Part print with two shaded views. Sizes in mm from the minimum x, y, z corner. Round coordinates to 2 decimals unless told otherwise and drop trailing zeros. Order: outer loops, then holes, each group sorted by start corner. A loop starts at its lowest first (then second) coordinate and runs counter-clockwise, first axis right, second up. Notation, with made-up numbers: M 61,76.5 L 97,76.5 A3 cw 97,81.5 Z; hole C 46,62 d10. An arc over 180 degrees is marked long. Return JSON: item names as keys, results as strings. Group by question number.
Item 1: Slice it at A-A on x = 18. Write the cut outline in (y, z).
Item 2: Slice it at D-D on z = 37. Write the cut outline in (x, y).
Item 3: Probe line 1 along X through (y, z) = (0.1, 21); line 2 along Z through (x, y) = (9.5, 0.2); line 3 along X through (y, z) = (0.3, 11). List the from-to ranges inside material, lowest first.
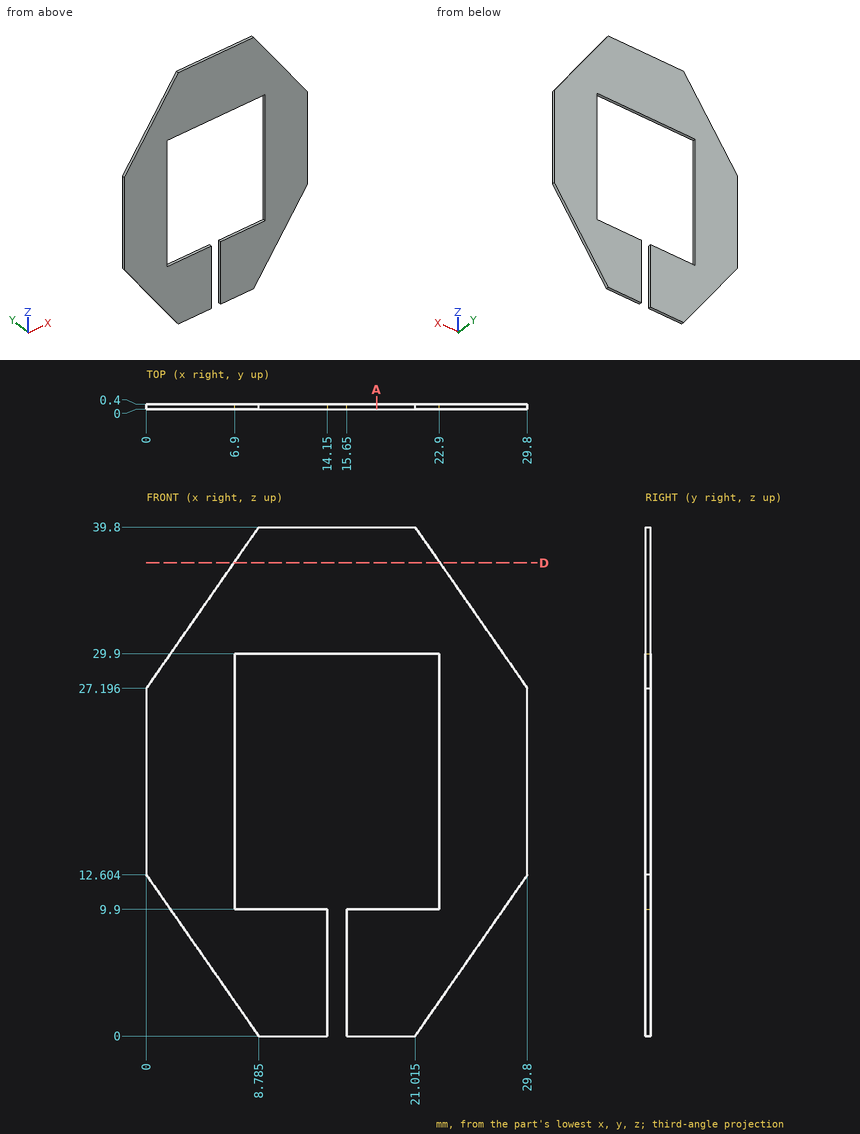
Output values:
{
 "1": {"outline": "M 0,0 L 0.4,0 L 0.4,9.9 L 0,9.9 Z; M 0,29.9 L 0.4,29.9 L 0.4,39.8 L 0,39.8 Z"},
 "2": {"outline": "M 6.83,0 L 22.97,0 L 22.97,0.4 L 6.83,0.4 Z"},
 "3": {"line 1": "0 to 6.9, 22.9 to 29.8", "line 2": "0 to 9.9, 29.9 to 39.8", "line 3": "1.12 to 6.9, 22.9 to 28.68"}
}
